Source: CAD feature listing. Evaluate the final solid. Frame: model axes, mm. A direction names the side the tool comes from. Give positions to 0.01 mm unless a question says otherwise; leave off trailing zeros. Loops run counter-clockwise (first coordinate to the right, second up) from the corner with the lowest first, then second, coordinate; pieces in that order, holes last.
Autodesk Inventor part; units mm, degrees
ref_plane "YZ Plane" through (0, 0, 0) normal (1, 0, 0) x (0, 1, 0)
ref_plane "XZ Plane" through (0, 0, 0) normal (0, 1, 0) x (-1, 0, 0)
ref_plane "XY Plane" through (0, 0, 0) normal (0, 0, 1) x (1, 0, 0)
sketch "Sketch1" plane through (0, 0, 0) normal (0, 1, 0) x (-1, 0, 0)
  line L0 (0, 0) -> (76.2, 0)
  line L1 (76.2, 0) -> (76.2, -76.2)
  line L2 (76.2, -76.2) -> (0, -76.2)
  line L3 (0, -76.2) -> (0, 0)
  dimension "d0" = 76.2
  dimension "d1" = 76.2
extrude "Extrusion1" add sketch "Sketch1" along normal blind 12.7
sketch "Sketch2" plane through (0, 12.7, 0) normal (0, 1, 0) x (1, 0, 0)
  point P0 (0, 0)
  point P1 (-12.7, 12.7)
  point P2 (-63.5, 12.7)
hole "Hole1" at (-12.7, 12.7, -12.7) at (-63.5, 12.7, -12.7) direction (0, -1, 0) diameter 5.08 depth 9.525 tip angle 118
sketch "Sketch3" plane through (0, 12.7, 0) normal (0, 1, 0) x (1, 0, 0)
  line L0 (0, 76.2) -> (-76.2, 76.2)
  line L1 (-44.45, 76.2) -> (-31.75, 76.2)
  line L2 (-31.75, 76.2) -> (-31.75, 63.5)
  line L3 (-31.75, 63.5) -> (-44.45, 63.5)
  line L4 (-44.45, 63.5) -> (-44.45, 76.2)
  point P0 (0, 0)
  point P1 (-38.1, 76.2)
  dimension "d11" = 12.7
  dimension "d12" = 12.7
extrude "Extrusion2" add sketch "Sketch3" along normal blind 25.4
sketch "Sketch4" plane through (0, 0, -76.2) normal (0, 0, -1) x (-1, 0, 0)
  point P0 (0, 0)
  point P1 (38.1, 31.75)
hole "Hole2" at (-38.1, 31.75, -76.2) direction (0, 0, 1) diameter 6.35 depth 14.2875 tip angle 118
fillet "Fillet1" radius 3.175 3 edges at (-31.75, 12.7, -69.85) (-38.1, 12.7, -63.5) (-44.45, 12.7, -69.85)
sketch "Sketch5" plane through (0, 12.7, 0) normal (0, 1, 0) x (1, 0, 0)
  circle A0 centre (-63.5, 12.7) radius 2.54
  point P0 (0, 0)
  point P1 (-12.7, 12.7)
hole "Hole3" at (-63.5, 12.7, -12.7) at (-12.7, 12.7, -12.7) direction (0, -1, 0) diameter 6.35 depth 9.525 tip angle 118
sketch "Sketch6" plane through (0, 12.7, 0) normal (0, 1, 0) x (1, 0, 0)
  circle A0 centre (-63.5, 12.7) radius 3.175
  circle A1 centre (-12.6652, 12.7) radius 3.2098
  circle A2 centre (-63.5, 12.7) radius 3.175
  point P0 (0, 0)
extrude "Extrusion3" add sketch "Sketch6" along normal blind 41.275 and the other way blind 12.7127
fillet "Fillet2" radius 3.175 1 edges at (-15.875, 12.7, -12.7)
fillet "Fillet3" radius 3.175 1 edges at (-66.675, 12.7, -12.7)
properties part number "Cupholder"
(1) Section B-B, the plane z = -69. Return the cut outline in (x, y) (3 decimals), then the cut area to 3 significant figures.
A:
outline: (-76.2, 0) - (0, 0) - (0, 12.7) - (-28.575, 12.7) arc R3.175 cw to (-31.75, 15.875) - (-31.75, 38.1) - (-44.45, 38.1) - (-44.45, 15.875) arc R3.175 cw to (-47.625, 12.7) - (-76.2, 12.7) - close; hole circle Ø6.35 at (-38.1, 31.75)
area: 1,260 mm2
(2) Section A-A, the plane x = -38.1. Return the cut outline in (y, z) (3 decimals).
A:
outline: (0, -76.2) - (28.575, -76.2) - (28.575, -63.5) - (15.875, -63.5) arc R3.175 cw to (12.7, -60.325) - (12.7, 0) - (0, 0) - close; (34.925, -76.2) - (38.1, -76.2) - (38.1, -63.5) - (34.925, -63.5) - close
(3) Mould query, pull axis X, two halves, no side actions, for faces 1 (the cylindrical face through (-60.57, 34.66, -13.92)), 2 (the flat face through (-13, -0.013, -13)), 3 (the cylindrical face through (-30.84, 13.65, -69.92)), 4 (the cylindrical face through (-40.777, 33.457, -69.761)). Classes: pulls with the +X half, pulls with the -X half, needs draft (parallel to the pull), parting line crosses it, or undercut.
A:
face 1: undercut
face 2: needs draft
face 3: pulls with the +X half
face 4: undercut
(4) Section D-D, the plane z = -12.7. Return the cut outline in (x, y) (3 decimals).
A:
outline: (-76.2, 0) - (-66.675, 0) - (-66.675, -0.013) - (-60.325, -0.013) - (-60.325, 0) - (-15.875, 0) - (-15.875, -0.013) - (-9.455, -0.013) - (-9.455, 0) - (0, 0) - (0, 12.7) - (-6.28, 12.7) arc R3.175 cw to (-9.455, 15.875) - (-9.455, 53.975) - (-15.875, 53.975) - (-15.875, 15.875) arc R3.175 cw to (-19.05, 12.7) - (-57.15, 12.7) arc R3.175 cw to (-60.325, 15.875) - (-60.325, 53.975) - (-66.675, 53.975) - (-66.675, 15.875) arc R3.175 cw to (-69.85, 12.7) - (-76.2, 12.7) - close
(5) First-contact query: pin 1 (6.5 mm diameter, centred on y = 26.5, z = -70.5, fed in from -X); pin 2 (10 mm diameter, centred on x = -60.5, z = -22.5, fed in from -Y); pin 3 (4 mm diameter, centred on x = -46, z = -46.5, fed in from +Y); pin 4 (6 mm diameter, centred on y = 37.5, z = -19.5, fed in from -X). Flat tips, straight axial feed; report the tip coordinate or a pass-through.
A:
pin 1: stops at x = -44.45
pin 2: stops at y = 0
pin 3: stops at y = 12.7
pin 4: passes through
(6) Section C-C, the plane y = 31.75. Return the cut outline in (x, z) (3 decimals), then the cut area to 3 significant figures.
A:
outline: circle Ø6.35 at (-63.5, -12.7); (-44.45, -76.2) - (-41.275, -76.2) - (-41.275, -63.5) - (-44.45, -63.5) - close; (-34.925, -76.2) - (-31.75, -76.2) - (-31.75, -63.5) - (-34.925, -63.5) - close; circle Ø6.42 at (-12.665, -12.7)
area: 145 mm2
(7) Ray query, line 1 along Y through (x, z) = (-38.1, -69) (3 decimals); line 2 along X through (y, z) = (31.75, -68.5) (3 decimals); line 3 along Z through (x, y) = (-43.5, 27). Return the intervals inside material, ascending.
A:
line 1: y = 0 to 28.575, 34.925 to 38.1
line 2: x = -44.45 to -41.275, -34.925 to -31.75
line 3: z = -76.2 to -63.5
(8) Reachability of faces 5 (the flat face through (-44.45, 27, -70)), 6 (the flat face through (-31.75, 27, -70)), 7 (the flat face through (-38, 27, -63.5)), 8 (the cylindrical face through (-11.184, 34.658, -15.548)) from +Z, -Z, +X, -X, +Y, -Y: full face, straight path, thin tool, end or side. Return the list, or none.
A:
face 5: +Z, -Z, -X, +Y
face 6: +Z, -Z, +X, +Y
face 7: +Z, +X, -X, +Y
face 8: +Y
